The model under review builds one solid part; all positions refer to its coordinate system, in mm. Round coordinates to 2 decimals unless told otherwise and drop trailing zeros. Order: outer loops, then holes, each group sorted by start corner. A loop starts at its lowest first (then second) coordinate and runs counter-clockwise, first axis right, second up. Notation, with made-up numbers: (36.25, -19) -> (59.25, -19) arc R25 cw to (59.25, 8) -> close; hole circle Ø11 at (4.25, 33.25). An arc over 180 degrees is marked (long way). Use a Markdown table: item, result. Add a question column.
```python
from build123d import *

# Parameters (mm, degrees)
F0_R          = 31.75
F1_DEPTH      = 76.2
F1_DEPTH_BACK = 76.2
F2_R          = 10.16
F3_SIZE       = 10.16


with BuildPart() as f1:
    # F0 (on Top) → F1 (new body, two sides)
    with BuildSketch(Plane.XY) as f1_sk:
        Circle(F0_R)
    extrude(amount=-F1_DEPTH)
    extrude(f1_sk.sketch, amount=F1_DEPTH_BACK)

    # F2
    f2_edges = [f1.edges().sort_by_distance(p)[0] for p in [
        (-31.75, 0, 76.2),
    ]]
    fillet(f2_edges, radius=F2_R)

    # F3
    f3_edges = [f1.edges().sort_by_distance(p)[0] for p in [
        (-31.75, 0, -76.2),
    ]]
    chamfer(f3_edges, length=F3_SIZE)


solid = f1.part
```
Q1. Add section A-A (y = 0). Write out the cut boundary in (x, z), then the cut area to 3 significant figures.
Q2. Wall thickness on line 1 (Y direction, x = 0.5, z = 0); line 2 (Y direction, x = -9, z = -44); line 3 (X direction, y = 16, z = -12): over which ranges is each line inside the solid? List them lowest first. Write a range as [from, to].
Q3. Insertion check: pin 1 (6 mm diameter, centred on y = -10.5, z = -21.5, fed in from -X); pin 2 (3 mm diameter, centred on x = -18, y = -24.5, fed in from +Z); pin 3 (5 mm diameter, centred on x = -5.5, z = 47, fed in from +Y). Each pin has a flat end and moves straight along its axis. Give the tip position at first contact, or say it passes through.
Q4. Add section C-C (z = 61.5). Write out the cut boundary in (x, y).
Report:
| question | item | result |
|---|---|---|
| 1 | outline | (-31.75, -66.04) -> (-21.59, -76.2) -> (21.59, -76.2) -> (31.75, -66.04) -> (31.75, 66.04) arc R10.16 ccw to (21.59, 76.2) -> (-21.59, 76.2) arc R10.16 ccw to (-31.75, 66.04) -> close |
| 1 | area | 9,530 mm² |
| 2 | line 1 | y = [-31.75, 31.75] |
| 2 | line 2 | y = [-30.45, 30.45] |
| 2 | line 3 | x = [-27.42, 27.42] |
| 3 | pin 1 | stops at x = -30.85 |
| 3 | pin 2 | stops at z = 73.09 |
| 3 | pin 3 | stops at y = 31.61 |
| 4 | outline | circle Ø63.5 at (0, 0) |
